The model under review builds one solid part; all positions refer to its coordinate system, in mm. Face numbers are marked on the shaded views. A direction names the side the tool comes from. Give positions to 0.01 mm unless a question says otherwise; leave off trailing zeros. Loops run counter-clockwise (first coordinate to the right, second up) from the corner with the lowest first, then second, coordinate; pieces in that order, holes last. Notation, with made-up numbers: M 18.5,52 L 63.5,52 A16 ccw 63.5,64 Z; hole C 55.5,36 d11. An arc over 180 degrees is marked long. Return JSON: item names as keys, results as strings.
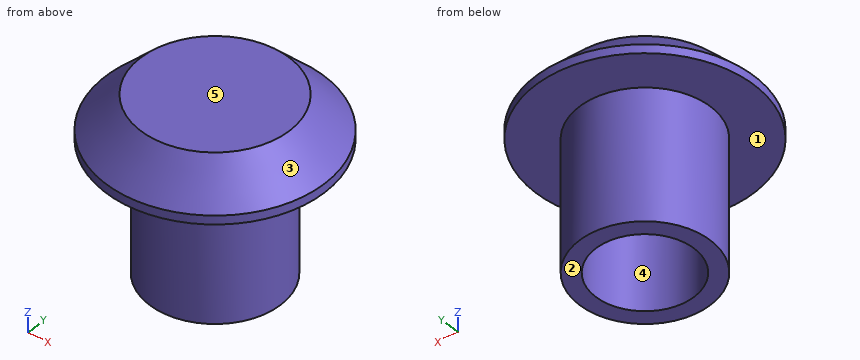
```python
from build123d import *

# Parameters (mm, degrees)
F0_R     = 15.875
F1_DEPTH = 6.35
F2_SIZE  = 5.08
F3_R     = 9.525
F3_R_2   = 7.14375
F4_DEPTH = 19.05


with BuildPart() as f1:
    # F0 (on Top) → F1 (new body)
    with BuildSketch(Plane.XY):
        Circle(F0_R)
    extrude(amount=F1_DEPTH)

    # F2
    f2_edges = [f1.edges().sort_by_distance(p)[0] for p in [
        (-15.875, 0, 6.35),
    ]]
    chamfer(f2_edges, length=F2_SIZE)

    # F3 (on face) → F4 (join)
    with BuildSketch(Plane(origin=(0, 0, 0), x_dir=(1, 0, 0), z_dir=(0, 0, -1))):
        Circle(F3_R)
        Circle(F3_R_2, mode=Mode.SUBTRACT)
    extrude(amount=F4_DEPTH)


solid = f1.part
```
1) Wall thickness on L1, parallel to X at y = 0, z = -14 (3 decimals); L2, parallel to Z at x = 2.5, y = 0.5: over which ranges is each line inside the solid? List them lowest first. Write a range as from..to.
From the geometry:
{"L1": "-9.525..-7.144, 7.144..9.525", "L2": "0..6.35"}
2) Insertion check: pin 1 (10 mm diameter, centred on x = 11, z = -9.5, fed in from +Y); pin 2 (3 mm diameter, centred on y = 12, z = 0, fed in from -X); pin 3 (1 mm diameter, centred on y = -12.5, z = 2.5, fed in from -X). Each pin has a flat end and moves straight along its axis. Give the tip position at first contact, or say it passes through.
From the geometry:
{"pin 1": "y = 7.4", "pin 2": "x = -11.91", "pin 3": "x = -8.8"}
3) Consider section A-A on x = 0. Write out the cut boundary in (y, z) (3 decimals), then the cut area to 3 significant figures.
From the geometry:
{"outline": "M -15.875,0 L -9.525,0 L -9.525,-19.05 L -7.144,-19.05 L -7.144,0 L 7.144,0 L 7.144,-19.05 L 9.525,-19.05 L 9.525,0 L 15.875,0 L 15.875,1.27 L 10.795,6.35 L -10.795,6.35 L -15.875,1.27 Z", "area": "267 mm²"}
4) Tool access review of the marked faces 1 and 2: name each direction out of +Z, -Z, +X, -X, +Y, -Y from which nothing blocks a thin tool from reaching the whole face with its end or side.
From the geometry:
{"face 1": "-Z", "face 2": "-Z, +X, -X, +Y, -Y"}
5) The part is to be moulded in two halves that separate along Y. For the marked faces 3, 4 and 5, say which applies: released by +Y, released by -Y, zero draft, split by the parting line, or undercut.
From the geometry:
{"face 3": "split by the parting line", "face 4": "undercut", "face 5": "zero draft"}
6) Consider section D-D on z = 4. Write out the cut boundary in (x, y) (3 decimals).
From the geometry:
{"outline": "C 0,0 d26.29"}
